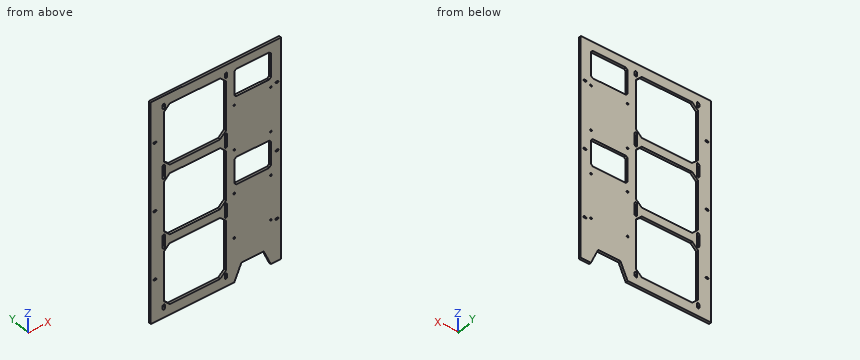
from build123d import *

# Parameters (mm, degrees)
SKETCH_1_R      = 1.45
EXTRUDE_1_DEPTH = 4


with BuildPart() as part:
    # 草圖1 → 填料-伸長1 (new body)
    with BuildSketch(Plane(origin=(0, 4, 0), x_dir=(1, 0, 0), z_dir=(0, 1, 0))):
        Polygon((110, 190.5), (92.72, 190.5), (80.72, 162.5), (43, 162.5), (31, 190.5), (-110, 190.5), (-110, -190.5), (110, -190.5), align=None)
        with Locations((31, 114.1)):
            Circle(SKETCH_1_R, mode=Mode.SUBTRACT)
        with Locations((92.72, 114.1)):
            Circle(SKETCH_1_R, mode=Mode.SUBTRACT)
        with Locations((31, 37.5)):
            Circle(SKETCH_1_R, mode=Mode.SUBTRACT)
        with Locations((92.72, 37.5)):
            Circle(SKETCH_1_R, mode=Mode.SUBTRACT)
        with Locations((31, -37.5)):
            Circle(SKETCH_1_R, mode=Mode.SUBTRACT)
        with Locations((92.72, -37.5)):
            Circle(SKETCH_1_R, mode=Mode.SUBTRACT)
        with Locations((31, -114.1)):
            Circle(SKETCH_1_R, mode=Mode.SUBTRACT)
        with Locations((92.72, -114.1)):
            Circle(SKETCH_1_R, mode=Mode.SUBTRACT)
        with BuildLine():
            Line((-104, 1.5), (-102, 1.5))
            ThreePointArc((-102, 1.5), (-100.5, 0), (-102, -1.5))
            Line((-102, -1.5), (-104, -1.5))
            ThreePointArc((-104, -1.5), (-105.5, 0), (-104, 1.5))
        make_face(mode=Mode.SUBTRACT)
        with BuildLine():
            Line((102, -116), (104, -116))
            ThreePointArc((104, -116), (105.5, -117.5), (104, -119))
            Line((104, -119), (102, -119))
            ThreePointArc((102, -119), (100.5, -117.5), (102, -116))
        make_face(mode=Mode.SUBTRACT)
        with BuildLine():
            Line((102, 1.5), (104, 1.5))
            ThreePointArc((104, 1.5), (105.5, 0), (104, -1.5))
            Line((104, -1.5), (102, -1.5))
            ThreePointArc((102, -1.5), (100.5, 0), (102, 1.5))
        make_face(mode=Mode.SUBTRACT)
        with BuildLine():
            Line((102, 119), (104, 119))
            ThreePointArc((104, 119), (105.5, 117.5), (104, 116))
            Line((104, 116), (102, 116))
            ThreePointArc((102, 116), (100.5, 117.5), (102, 119))
        make_face(mode=Mode.SUBTRACT)
        with BuildLine():
            Line((-104, -116), (-102, -116))
            ThreePointArc((-102, -116), (-100.5, -117.5), (-102, -119))
            Line((-102, -119), (-104, -119))
            ThreePointArc((-104, -119), (-105.5, -117.5), (-104, -116))
        make_face(mode=Mode.SUBTRACT)
        with BuildLine():
            Line((-104, 119), (-102, 119))
            ThreePointArc((-102, 119), (-100.5, 117.5), (-102, 116))
            Line((-102, 116), (-104, 116))
            ThreePointArc((-104, 116), (-105.5, 117.5), (-104, 119))
        make_face(mode=Mode.SUBTRACT)
        with BuildLine():
            Line((-90, -175.1), (-90, -169.9))
            ThreePointArc((-90, -169.9), (-88, -167.9), (-86, -169.9))
            Line((-86, -169.9), (-86, -175.1))
            ThreePointArc((-86, -175.1), (-88, -177.1), (-90, -175.1))
        make_face(mode=Mode.SUBTRACT)
        with BuildLine():
            Line((15, -70.1), (15, -49.9))
            ThreePointArc((15, -49.9), (17, -47.9), (19, -49.9))
            Line((19, -49.9), (19, -70.1))
            ThreePointArc((19, -70.1), (17, -72.1), (15, -70.1))
        make_face(mode=Mode.SUBTRACT)
        with BuildLine():
            Line((-90, -70.1), (-90, -49.9))
            ThreePointArc((-90, -49.9), (-88, -47.9), (-86, -49.9))
            Line((-86, -49.9), (-86, -70.1))
            ThreePointArc((-86, -70.1), (-88, -72.1), (-90, -70.1))
        make_face(mode=Mode.SUBTRACT)
        with BuildLine():
            Line((19, 175.1), (19, 169.9))
            ThreePointArc((19, 169.9), (17, 167.9), (15, 169.9))
            Line((15, 169.9), (15, 175.1))
            ThreePointArc((15, 175.1), (17, 177.1), (19, 175.1))
        make_face(mode=Mode.SUBTRACT)
        Polygon((89.72, -23.5), (34, -23.5), (31, -20.5), (31, 20.5), (34, 23.5), (89.72, 23.5), (92.72, 20.5), (92.72, -20.5), align=None, mode=Mode.SUBTRACT)
        Polygon((89.72, -175.1), (34, -175.1), (31, -172.1), (31, -131.1), (34, -128.1), (89.72, -128.1), (92.72, -131.1), (92.72, -172.1), align=None, mode=Mode.SUBTRACT)
        Polygon((-78, -172.5), (-88, -162.5), (-88, -77.5), (-78, -67.5), (7, -67.5), (17, -77.5), (17, -162.5), (7, -172.5), align=None, mode=Mode.SUBTRACT)
        Polygon((-78, -52.5), (-88, -42.5), (-88, 42.5), (-78, 52.5), (7, 52.5), (17, 42.5), (17, -42.5), (7, -52.5), align=None, mode=Mode.SUBTRACT)
        with BuildLine():
            Line((-86, 70.1), (-86, 49.9))
            ThreePointArc((-86, 49.9), (-88, 47.9), (-90, 49.9))
            Line((-90, 49.9), (-90, 70.1))
            ThreePointArc((-90, 70.1), (-88, 72.1), (-86, 70.1))
        make_face(mode=Mode.SUBTRACT)
        with BuildLine():
            Line((19, 70.1), (19, 49.9))
            ThreePointArc((19, 49.9), (17, 47.9), (15, 49.9))
            Line((15, 49.9), (15, 70.1))
            ThreePointArc((15, 70.1), (17, 72.1), (19, 70.1))
        make_face(mode=Mode.SUBTRACT)
        with BuildLine():
            Line((19, -169.9), (19, -175.1))
            ThreePointArc((19, -175.1), (17, -177.1), (15, -175.1))
            Line((15, -175.1), (15, -169.9))
            ThreePointArc((15, -169.9), (17, -167.9), (19, -169.9))
        make_face(mode=Mode.SUBTRACT)
        with BuildLine():
            Line((-86, 175.1), (-86, 169.9))
            ThreePointArc((-86, 169.9), (-88, 167.9), (-90, 169.9))
            Line((-90, 169.9), (-90, 175.1))
            ThreePointArc((-90, 175.1), (-88, 177.1), (-86, 175.1))
        make_face(mode=Mode.SUBTRACT)
        Polygon((17, 162.5), (17, 77.5), (7, 67.5), (-78, 67.5), (-88, 77.5), (-88, 162.5), (-78, 172.5), (7, 172.5), align=None, mode=Mode.SUBTRACT)
    extrude(amount=-EXTRUDE_1_DEPTH)


solid = part.part
Source: CAD feature listing. Evaluate the final solid. Frame: model axes, mm. Give positions to 0.01 mm unless a question says otherwise; leave off trailing zeros. Order: outer loops, then holes, each group sorted by start corner. A loop starts at its lowest first (then second) coordinate and runs counter-clockwise, first axis right, second up. Notation, with made-up numbers: (78.25, -25.75) -> (111.25, -25.75) arc R14 cw to (111.25, -4.75) -> close; hole circle Ø6 at (53.25, 81.25). An arc over 180 degrees is marked (long way). Write item = value, one per line.
Item 1: Section query B-B (x = -53). Output: boundary loops of the cut face in (y, z), then the cut area to 3 significant figures.
Check result:
outline = (0, -190.5) -> (4, -190.5) -> (4, -172.5) -> (0, -172.5) -> close; (0, -67.5) -> (4, -67.5) -> (4, -52.5) -> (0, -52.5) -> close; (0, 52.5) -> (4, 52.5) -> (4, 67.5) -> (0, 67.5) -> close; (0, 172.5) -> (4, 172.5) -> (4, 190.5) -> (0, 190.5) -> close
area = 264 mm²
Item 2: Section query A-A (z = 144). Output: boundary loops of the cut face in (x, y), then the cut area to 3 significant figures.
Check result:
outline = (-110, 0) -> (-88, 0) -> (-88, 4) -> (-110, 4) -> close; (17, 0) -> (31, 0) -> (31, 4) -> (17, 4) -> close; (92.72, 0) -> (110, 0) -> (110, 4) -> (92.72, 4) -> close
area = 213 mm²
Item 3: Ray query, probe 1 along X at (y, z) = (1.3, -37.5); probe 2 along Z at (x, y) = (-71, 1.65); probe 3 along X at (y, z) = (1.65, -59.5). Return the intervals inside material, ascending.
Check result:
probe_1 = -110 to -88, 17 to 29.55, 32.45 to 91.27, 94.17 to 110
probe_2 = -190.5 to -172.5, -67.5 to -52.5, 52.5 to 67.5, 172.5 to 190.5
probe_3 = -110 to -90, -86 to 15, 19 to 110
Item 4: Section query C-C (y = 1.4). State how many separate pieces and enclosed holes the cut face has, then the cut area to 3 significant figures.
Check result:
separate_pieces = 1
enclosed_holes = 27
area = 43,500 mm²
Item 5: Contact query for a flat-ended pin moving along its axis: pin 1 (2.5 mm diameter, centred on x = 31, z = -37.5, fed in from -Y). Output: stop coordinate, or through.
Check result:
pin_1 = through
